Input: part model. Units: mm. Frame: model coordinates. Give positions to 0.01 mm unless a question says otherwise; leave off trailing zeros. Loops run counter-clockwise (first coordinate to the right, second up) from the corner with the lowest first, then second, coordinate; pieces in that order, holes last. Notation, with made-up numbers: M 35,48.5 L 56,48.5 A26 ccw 56,65.5 Z; hole C 56,63 d4. An arc over 180 degrees is marked long. One line per item, written item: value. Start each with the question number.
(1) Section D-D on x = 50. Output: boundary loops of the cut face in (y, z), plus the area to 3 significant figures.
(2) Pin query (flat end, axial travel): P1, Ø5, axis at x = 115.21, y = 179, coming from the +Z side; P2, Ø10, axis at x = 175, y = 136.75, coming from the +Z side. Return the tip coordinate at first contact, or that it passes through.
(3) Section A-A on x = 200. Output: boundary loops of the cut face in (y, z) (3 decimals), plus the area to 3 significant figures.
(4) Section C-C on z = 16. State how many separate pieces and enclosed holes the cut face has, plus the area to 3 significant figures.
(5) Section B-B on y = 17.5. Output: boundary loops of the cut face in (x, z) (3 decimals).
(6) Ray query, line 1 along X through (y, z) = (17, 44); line 2 along Y through (x, z) = (50, 31.5); line 3 along Y through (x, z) = (114, 17). Return the intervals inside material, ascending. Write a range as from..to.
```python
from build123d import *

# Parameters (mm, degrees)
SKETCH1_W           = 300
SKETCH1_H           = 275
SKETCH1_R           = 12.7
SKETCH1_R_2         = 4.675
SKETCH1_R_3         = 3
BOSS_EXTRUDE1_DEPTH = 74
SKETCH2_R           = 6.35
CUT_EXTRUDE1_DEPTH  = 45


with BuildPart() as part:
    # Sketch1 → Boss-Extrude1 (new body)
    with BuildSketch(Plane.XY):
        with Locations((150, 137.5)):
            Rectangle(SKETCH1_W, SKETCH1_H)
        with Locations((250, 17.5)):
            Circle(SKETCH1_R, mode=Mode.SUBTRACT)
        with Locations((200, 17.5)):
            Circle(SKETCH1_R_2, mode=Mode.SUBTRACT)
        with Locations((100, 17.5)):
            Circle(SKETCH1_R_2, mode=Mode.SUBTRACT)
        with Locations((50, 17.5)):
            Circle(SKETCH1_R, mode=Mode.SUBTRACT)
        with Locations((235.25, 136.75)):
            Circle(SKETCH1_R_3, mode=Mode.SUBTRACT)
        with Locations((114.75, 136.75)):
            Circle(SKETCH1_R_3, mode=Mode.SUBTRACT)
        with Locations((175, 136.75)):
            Circle(SKETCH1_R_3, mode=Mode.SUBTRACT)
        with Locations((115.210881667, 178.997486175)):
            Circle(SKETCH1_R_3, mode=Mode.SUBTRACT)
        with Locations((175.307264601, 178.998882689)):
            Circle(SKETCH1_R_3, mode=Mode.SUBTRACT)
        with Locations((235.403635348, 178.999720664)):
            Circle(SKETCH1_R_3, mode=Mode.SUBTRACT)
    extrude(amount=BOSS_EXTRUDE1_DEPTH)

    # Sketch2 → Cut-Extrude1 (cut)
    with BuildSketch(Plane(origin=(0, 0, 74), x_dir=(-1, 0, 0), z_dir=(0, 0, -1))):
        with Locations((-175, 136.75)):
            Circle(SKETCH2_R)
        with Locations((-235.25, 136.75)):
            Circle(SKETCH2_R)
        with Locations((-235.403635348, 178.999720664)):
            Circle(SKETCH2_R)
        with Locations((-175.307264601, 178.998882689)):
            Circle(SKETCH2_R)
        with Locations((-115.210881667, 178.997486175)):
            Circle(SKETCH2_R)
        with Locations((-114.75, 136.75)):
            Circle(SKETCH2_R)
    extrude(amount=CUT_EXTRUDE1_DEPTH, mode=Mode.SUBTRACT)


solid = part.part
```
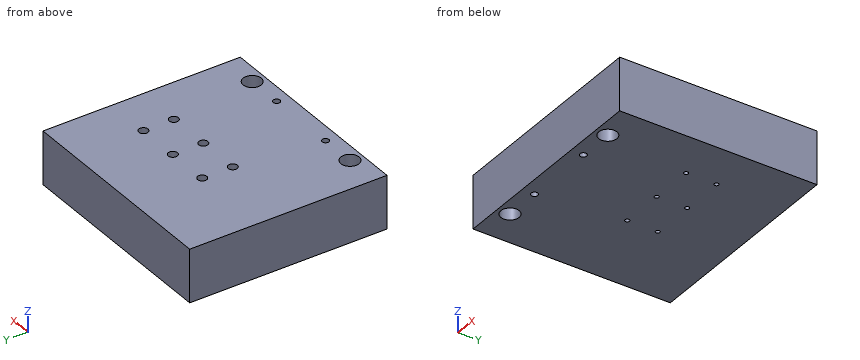
Output values:
1. outline: M 0,0 L 4.8,0 L 4.8,74 L 0,74 Z; M 30.2,0 L 275,0 L 275,74 L 30.2,74 Z
1. area: 18,500 mm²
2. P1: passes through
2. P2: stops at z = 29
3. outline: M 0,0 L 12.825,0 L 12.825,74 L 0,74 Z; M 22.175,0 L 275,0 L 275,74 L 22.175,74 Z
3. area: 19,700 mm²
4. separate pieces: 1
4. enclosed holes: 10
4. area: 81,200 mm²
5. outline: M 0,0 L 37.3,0 L 37.3,74 L 0,74 Z; M 62.7,0 L 95.325,0 L 95.325,74 L 62.7,74 Z; M 104.675,0 L 195.325,0 L 195.325,74 L 104.675,74 Z; M 204.675,0 L 237.3,0 L 237.3,74 L 204.675,74 Z; M 262.7,0 L 300,0 L 300,74 L 262.7,74 Z
6. line 1: x = 0..37.31, 62.69..95.35, 104.65..195.35, 204.65..237.31, 262.69..300
6. line 2: y = 0..4.8, 30.2..275
6. line 3: y = 0..133.85, 139.65..176.25, 181.74..275
